from build123d import *

# Parameters (mm, degrees)
F1_W         = 90.5
F1_H         = 90.5
F1_W_2       = 22
F1_H_2       = 22
F2_DEPTH     = 40
F4_DEPTH     = 0.6
F5_T1_DEPTH  = 40
F5_T6_DEPTH  = 64.4
F5_T11_DEPTH = 64.4
F6_R         = 10.5


# Not quite as in the source:
# - a fillet or chamfer that OpenCascade refuses, or shapes differently, is made with other operations: its cross-section is extruded or revolved along the edge and cut away or added


with BuildPart() as f2:
    # F1 (on Top) → F2 (new body)
    with BuildSketch(Plane.XY):
        with Locations((44.75, 44.75)):
            Rectangle(F1_W, F1_H)
        with Locations((11, 11)):
            Rectangle(F1_W_2, F1_H_2, mode=Mode.SUBTRACT)
        with Locations((33.5, 11)):
            Rectangle(F1_W_2, F1_H_2, mode=Mode.SUBTRACT)
        with Locations((11, 33.5)):
            Rectangle(F1_W_2, F1_H_2, mode=Mode.SUBTRACT)
        with Locations((33.5, 33.5)):
            Rectangle(F1_W_2, F1_H_2, mode=Mode.SUBTRACT)
        with Locations((56, 11)):
            Rectangle(F1_W_2, F1_H_2, mode=Mode.SUBTRACT)
        with Locations((78.5, 11)):
            Rectangle(F1_W_2, F1_H_2, mode=Mode.SUBTRACT)
        with Locations((56, 33.5)):
            Rectangle(F1_W_2, F1_H_2, mode=Mode.SUBTRACT)
        with Locations((78.5, 33.5)):
            Rectangle(F1_W_2, F1_H_2, mode=Mode.SUBTRACT)
        with Locations((11, 56)):
            Rectangle(F1_W_2, F1_H_2, mode=Mode.SUBTRACT)
        with Locations((33.5, 56)):
            Rectangle(F1_W_2, F1_H_2, mode=Mode.SUBTRACT)
        with Locations((11, 78.5)):
            Rectangle(F1_W_2, F1_H_2, mode=Mode.SUBTRACT)
        with Locations((33.5, 78.5)):
            Rectangle(F1_W_2, F1_H_2, mode=Mode.SUBTRACT)
        with Locations((56, 56)):
            Rectangle(F1_W_2, F1_H_2, mode=Mode.SUBTRACT)
        with Locations((78.5, 56)):
            Rectangle(F1_W_2, F1_H_2, mode=Mode.SUBTRACT)
        with Locations((56, 78.5)):
            Rectangle(F1_W_2, F1_H_2, mode=Mode.SUBTRACT)
        with Locations((78.5, 78.5)):
            Rectangle(F1_W_2, F1_H_2, mode=Mode.SUBTRACT)
    extrude(amount=F2_DEPTH)

    # F3 (on face) → F4 (join)
    with BuildSketch(Plane(origin=(0, 0, 0), x_dir=(1, 0, 0), z_dir=(0, 0, -1))):
        Polygon((22, -89.5), (22, -88.0857864376), (1.4142135624, -67.5), (0, -67.5), (0, -68.9142135624), (20.5857864376, -89.5), align=None)
        Polygon((22, -67), (22, -65.5857864376), (1.4142135624, -45), (0, -45), (0, -46.4142135624), (20.5857864376, -67), align=None)
        Polygon((44.5, -89.5), (44.5, -88.0857864376), (23.9142135624, -67.5), (22.5, -67.5), (22.5, -68.9142135624), (43.0857864376, -89.5), align=None)
        Polygon((22, -44.5), (22, -43.0857864376), (1.4142135624, -22.5), (0, -22.5), (0, -23.9142135624), (20.5857864376, -44.5), align=None)
        Polygon((44.5, -67), (44.5, -65.5857864376), (23.9142135624, -45), (22.5, -45), (22.5, -46.4142135624), (43.0857864376, -67), align=None)
        Polygon((67, -89.5), (67, -88.0857864376), (46.4142135624, -67.5), (45, -67.5), (45, -68.9142135624), (65.5857864376, -89.5), align=None)
        Polygon((89.5, -89.5), (89.5, -88.0857864376), (68.9142135624, -67.5), (67.5, -67.5), (67.5, -68.9142135624), (88.0857864376, -89.5), align=None)
        Polygon((67, -67), (67, -65.5857864376), (46.4142135624, -45), (45, -45), (45, -46.4142135624), (65.5857864376, -67), align=None)
        Polygon((44.5, -44.5), (44.5, -43.0857864376), (23.9142135624, -22.5), (22.5, -22.5), (22.5, -23.9142135624), (43.0857864376, -44.5), align=None)
        Polygon((22, -22), (22, -20.5857864376), (1.4142135624, 0), (0, 0), (0, -1.4142135624), (20.5857864376, -22), align=None)
        Polygon((22.5, -1.4142135624), (43.0857864376, -22), (44.5, -22), (44.5, -20.5857864376), (23.9142135624, 0), (22.5, 0), align=None)
        Polygon((45, -23.9142135624), (65.5857864376, -44.5), (67, -44.5), (67, -43.0857864376), (46.4142135624, -22.5), (45, -22.5), align=None)
        Polygon((67.5, -46.4142135624), (88.0857864376, -67), (89.5, -67), (89.5, -65.5857864376), (68.9142135624, -45), (67.5, -45), align=None)
        Polygon((67.5, -23.9142135624), (88.0857864376, -44.5), (89.5, -44.5), (89.5, -43.0857864376), (68.9142135624, -22.5), (67.5, -22.5), align=None)
        Polygon((45, -1.4142135624), (65.5857864376, -22), (67, -22), (67, -20.5857864376), (46.4142135624, 0), (45, 0), align=None)
        Polygon((67.5, -1.4142135624), (88.0857864376, -22), (89.5, -22), (89.5, -20.5857864376), (68.9142135624, 0), (67.5, 0), align=None)
    extrude(amount=-F4_DEPTH)

    # F5: fillet of radius 10 on 4 edges, made by hand

    # F5_s2 → F5_t1 (join)
    with BuildSketch(Plane.XY):
        with BuildLine():
            ThreePointArc((89.5, 10), (86.5710678119, 2.9289321881), (79.5, 0))
            Line((79.5, 0), (89.5, 0))
            Line((89.5, 0), (89.5, 10))
        make_face()
        with BuildLine():
            ThreePointArc((10, 89.5), (2.9289321881, 86.5710678119), (0, 79.5))
            Line((0, 79.5), (0, 89.5))
            Line((0, 89.5), (10, 89.5))
        make_face()
    extrude(amount=F5_T1_DEPTH)


with BuildPart() as f5_tool4:
    # F5_s5 → F5_t6 (new body)
    with BuildSketch(Plane.XY.offset(-24.4)):
        with BuildLine():
            ThreePointArc((0, 10), (2.9289321881, 2.9289321881), (10, 0))
            Line((10, 0), (0, 0))
            Line((0, 0), (0, 10))
        make_face()
    extrude(amount=F5_T6_DEPTH)

    split(bisect_by=Plane.XY, keep=Keep.TOP)


with BuildPart() as f2_1:
    add(f2.part)

    # F5_t3: union F5_tool4
    add(f5_tool4.part)


with BuildPart() as f5_tool9:
    # F5_s10 → F5_t11 (new body)
    with BuildSketch(Plane.XY.offset(-24.4)):
        with BuildLine():
            ThreePointArc((79.5, 89.5), (86.5710678119, 86.5710678119), (89.5, 79.5))
            Line((89.5, 79.5), (89.5, 89.5))
            Line((89.5, 89.5), (79.5, 89.5))
        make_face()
    extrude(amount=F5_T11_DEPTH)

    split(bisect_by=Plane.XY, keep=Keep.TOP)


with BuildPart() as f2_2:
    add(f2_1.part)

    # F5_t8: union F5_tool9
    add(f5_tool9.part)

    # F6
    f6_edges = [f2_2.edges().sort_by_distance(p)[0] for p in [
        (90, -0.5, 20),
        (-0.5, -0.5, 20),
        (-0.5, 90, 20),
        (90, 90, 20),
    ]]
    fillet(f6_edges, radius=F6_R)


solid = f2_2.part
Could you check a few things on this model? Use its own coordinates, in mm. A direction names the side the tool comes from. Give positions to 0.01 mm unless a question says otherwise; leave off trailing zeros. One line per question, with ' | ' between items. Start each with the question number.
Item 1: I need wall thicknesses on probe 1 along X at (y, z) = (77.5, 16); probe 2 along Y at (x, z) = (8, 8.5). Which ranges of each line are inside material? Lowest first, please. Write a range as [from, to].
Item 2: Thinking about a two-plate mould opening in Y: for faces 3 (the cylindrical face through (86.84, 87.01, 20.28)), 4 (the flat face through (33, 67, 20)), which applies, pulls with the +Y half, pulls with the -Y half, needs draft (parallel to the pull), parting line crosses it, or undercut?
Item 3: For faces 1 (the flat face through (55.149, 34.063, 0.296)), 2 (the flat face through (56, 33, 0.6)), which set-ups out of +Z, -Z, +X, -X, +Y, -Y let a thin tool reach every point of the face, with its end or its side?
Item 4: I'm going to push flat-ended pins straight in: pin 1 Ø11 at (x, y) = (61, 78.5) entering from +Z; pin 2 Ø1 at (x, y) = (43.5, 25.5) entering from -Z. Where does each tip first touch, or does it pass through?
Item 5: I want a section at A-A on z = 33. Give the number of separate pieces and of enclosed holes in the cut face, then the cut area to 3 significant figures.
Verdict:
1) probe 1: [-0.5, 0], [22, 22.5], [44.5, 45], [67, 67.5], [89.5, 90] | probe 2: [-0.31, 0.2], [22, 22.5], [44.5, 45], [67, 67.5], [89.3, 89.81]
2) face 3: pulls with the +Y half | face 4: undercut
3) face 1: +Z, -Z | face 2: +Z
4) pin 1: z = 0.6 | pin 2: through
5) separate pieces: 1 | enclosed holes: 16 | area: 437 mm^2
